For this review, use the dimensioned drawing (mm, ordinates from the lowest corner) and the shaded views. Round coordinates to 2 decimals unless told otherwise and drop trailing zeros. Order: outer loops, then holes, each group sorted by start corner. A loop starts at its lowest first (then second) coordinate and runs counter-clockwise, first axis right, second up. Notation, with made-up numbers: (21, 63.25) - (78, 63.25) arc R35 cw to (78, 102.25) - close; hole circle Ø1 at (63.25, 78). An arc over 180 degrees is marked (long way). Write item = value, one per line.
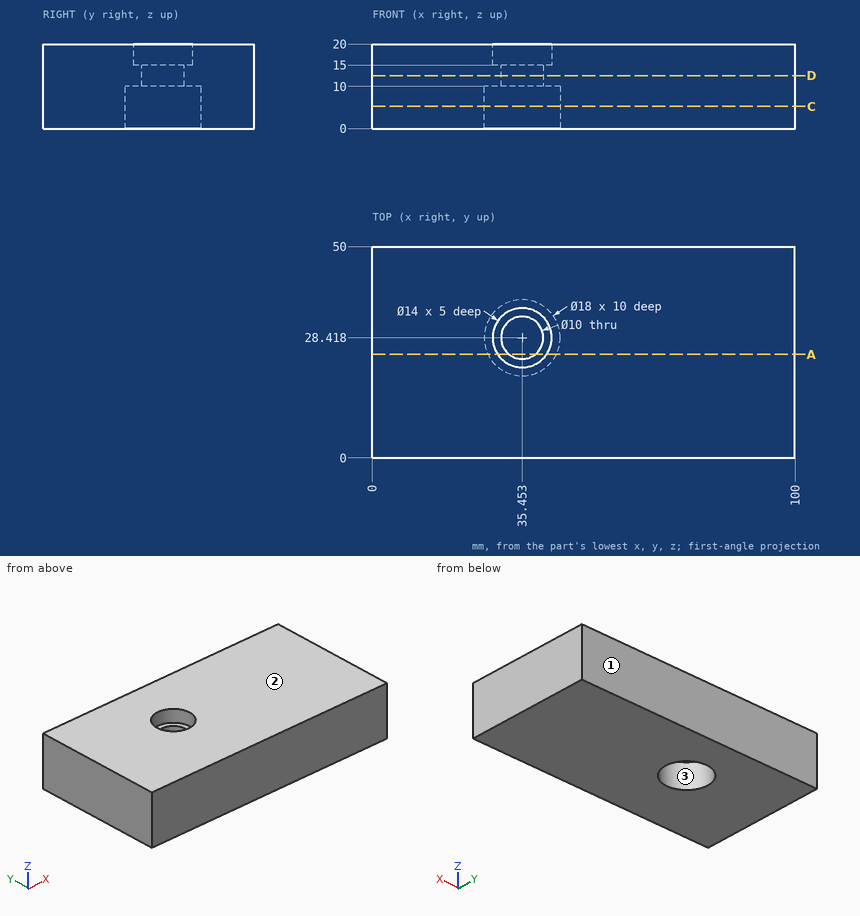
1) We need section C-C on z = 5.25. Write out the cut boundary in (x, y).
Findings:
outline = (0, 0) - (100, 0) - (100, 50) - (0, 50) - close; hole circle Ø18 at (35.45, 28.42)
2) To check wall thickness, follow L1, parallel to X at y = 23, z = 5.25 (1 decimal); L2, parallel to Y at x = 41, z = 8.5 (1 decimal); L3, parallel to Y at x = 32.5, z = 15.25 (1 decimal). State the ranges of each line that lie inside material, in increasing order. Write a range as from..to.
Findings:
L1 = 0..28.3, 42.6..100
L2 = 0..21.3, 35.5..50
L3 = 0..22.1, 34.8..50
3) We need section D-D on z = 12.5. Write out the cut boundary in (x, y).
Findings:
outline = (0, 0) - (100, 0) - (100, 50) - (0, 50) - close; hole circle Ø10 at (35.45, 28.42)
4) The part is to be moulded in two halves that separate along Y. For the marked faces 1, 2 and 3, say which applies: released by +Y, released by -Y, zero draft, split by the parting line, or undercut.
Findings:
face_1 = released by +Y
face_2 = zero draft
face_3 = undercut
5) Clearance check with flat-ended pins moving along their axes: pin 1 Ø7 at (x, y) = (35.5, 31) entering from +Z; pin 2 Ø4 at (x, y) = (45, 28) entering from -Z; pin 3 Ø5.5 at (x, y) = (32, 28.5) entering from -Z. State where each tip first meets the part, or that it passes through.
Findings:
pin_1 = 15
pin_2 = 0
pin_3 = 10
6) We need section A-A on y = 24.5. Write out the cut boundary in (x, z).
Findings:
outline = (0, 0) - (27.35, 0) - (27.35, 10) - (32.35, 10) - (32.35, 15) - (29.65, 15) - (29.65, 20) - (0, 20) - close; (38.56, 10) - (43.56, 10) - (43.56, 0) - (100, 0) - (100, 20) - (41.25, 20) - (41.25, 15) - (38.56, 15) - close
